Can you work these out from the drawing? Everything is in mm from the part's minimum corner. Coordinates: 2 decimals unless noted, no trailing zeros. Loops run counter-clockwise (first coordinate to the right, second up) from the corner with the lowest first, then second, coordinate; pieces in that order, holes last.
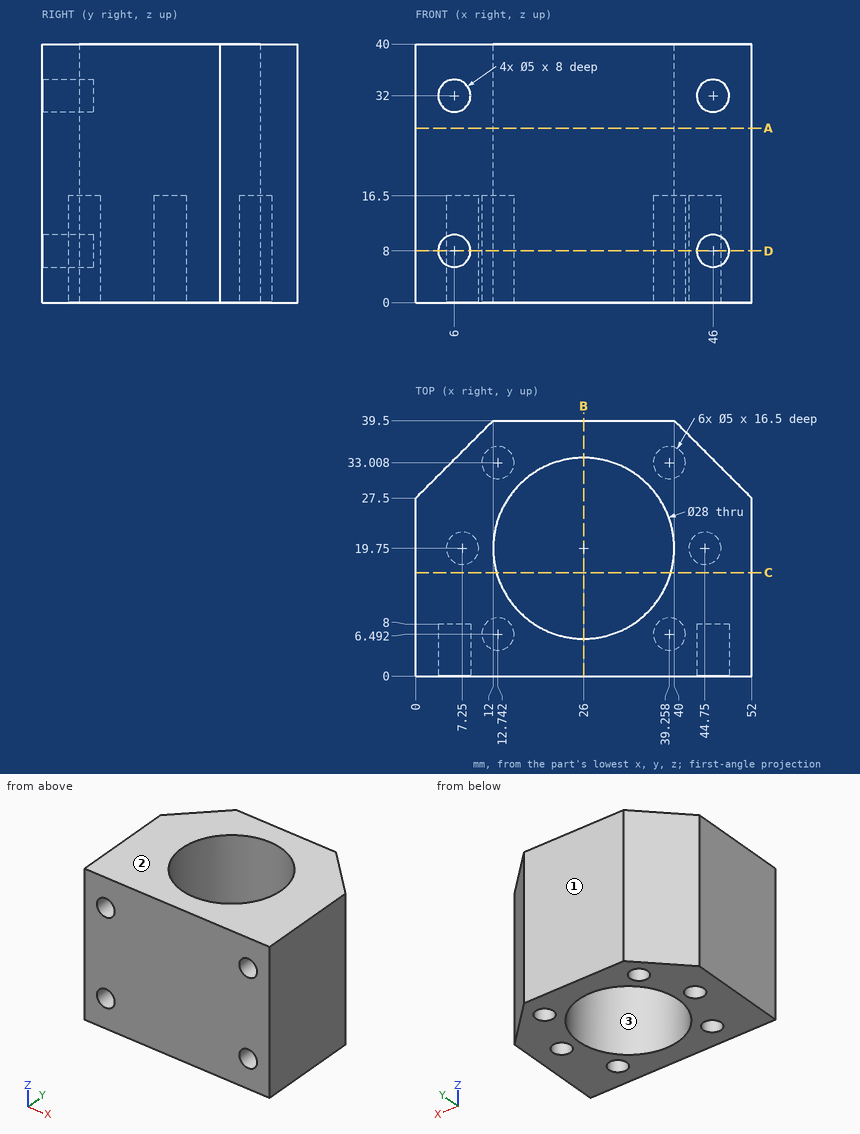
(1) We'd pull the mould along Y, two halves only. Please class the marked faces 1, 2 and 3: +Y half, -Y half, draft (parallel to the pull), parting line (faces both ways), or undercut.
Answers:
face 1: +Y half
face 2: draft
face 3: undercut
(2) Imagine slicing it at B-B, the plane x = 26. Write out the boundary of the cut face in (y, z), and give its area (3 significant figures).
Answers:
outline: (0, 0) - (5.75, 0) - (5.75, 40) - (0, 40) - close; (33.75, 0) - (39.5, 0) - (39.5, 40) - (33.75, 40) - close
area: 460 mm2
(3) Imagine slicing it at A-A, the plane z = 27. Write out the boundary of the cut face in (x, y), and give its area (3 significant figures).
Answers:
outline: (0, 0) - (52, 0) - (52, 27.5) - (40, 39.5) - (12, 39.5) - (0, 27.5) - close; hole circle Ø28 at (26, 19.75)
area: 1,290 mm2
(4) For pin 1 (2.5 mm diameter, centred on x = 45.5, y = 20.5, fed in from -Z); pin 2 (6 mm diameter, centred on x = 13, z = 33.5, fed in from -Y); pin 3 (3 mm diameter, centred on x = 46, z = 8, fed in from +Y); pin 4 (22.5 mm diameter, centred on x = 26, y = 19.75, fed in from +Z), each with a flat end and sliding along its axis, tell me the tip position at first contact or that it passes through.
Answers:
pin 1: stops at z = 16.5
pin 2: stops at y = 0
pin 3: stops at y = 35
pin 4: passes through
(5) Imagine slicing it at D-D, the plane z = 8. Write out the boundary of the cut face in (x, y).
Answers:
outline: (0, 0) - (3.5, 0) - (3.5, 8) - (8.5, 8) - (8.5, 0) - (43.5, 0) - (43.5, 8) - (48.5, 8) - (48.5, 0) - (52, 0) - (52, 27.5) - (40, 39.5) - (12, 39.5) - (0, 27.5) - close; hole circle Ø5 at (7.25, 19.75); hole circle Ø5 at (12.74, 6.49); hole circle Ø5 at (12.74, 33.01); hole circle Ø28 at (26, 19.75); hole circle Ø5 at (39.26, 6.49); hole circle Ø5 at (39.26, 33.01); hole circle Ø5 at (44.75, 19.75)
(6) I need wall thicknesses on probe 1 along X at (y, z) = (2, 32); probe 2 along X at (y, z) = (8.5, 4); probe 3 along Y at (x, z) = (26, 27). Which ranges of each line are inside material? Lowest first, please.
Answers:
probe 1: x = 0 to 3.5, 8.5 to 43.5, 48.5 to 52
probe 2: x = 0 to 11.25, 14.23 to 17.67, 34.33 to 37.77, 40.75 to 52
probe 3: y = 0 to 5.75, 33.75 to 39.5
(7) Imagine slicing it at C-C, the plane y = 16. Write out the boundary of the cut face in (x, z), and give its area (3 significant figures).
Answers:
outline: (0, 0) - (12.51, 0) - (12.51, 40) - (0, 40) - close; (39.49, 0) - (52, 0) - (52, 40) - (39.49, 40) - close
area: 1,000 mm2
